Part model, mm, in its own coordinate system. A direction names the side the tool comes from. Round coordinates to 2 decimals unless told otherwise and drop trailing zeros. Write each question's results on one line, items separated by ' | '. Start each with the question number.
(1) Drill centre lines: L1, parallel to Z at x = 9.5, y = 10.15; L2, parallel to X at y = 7, z = 9.5; L3, parallel to X at y = -5.5, z = 13.25. Where is each one in solid material? Low to high.
(2) Tool access for faces 1 (the face through (7, 7, 24)), 2 (the face through (8.2, 3.5, 13.4)), 3 (the face through (5.137, -4.644, 14.37)), 4 (the face through (11.452, 11.451, 18.566)): list every direction of +Z, -Z, +X, -X, +Y, -Y with a clear straight run to the whole face (end or side of a thin tool).
(3) Flat gauge pins, fed straight in: P1, Ø6, axis at x = 9.5, z = 12, coming from the -Y side; P2, Ø5, axis at x = 0, y = 7, coming from the +Z side; P3, Ø2, axis at y = -5, z = 11, coming from the -X side; P4, Ø4, axis at x = 9.5, z = 12, coming from the -Y side. Where does each tip first touch, or does it go through?
(4) Mould opens along Y. For faces 5 (the face through (5.137, -1.856, 9.63)), 6 (the face through (-3.2, -8.5, 12.1)), 7 (the face through (11, 10, 12.8)), 8 (the face through (6, 14, 12)) say: released by +Y, released by -Y, zero draft, split by the parting line, or undercut.
(5) Cut at B-B, the plane x = -1.75. Give the number of separate pieces and of enclosed holes in the cut face, then the cut area to 3 significant figures.
Autodesk Inventor part; units mm, degrees
ref_plane "Work Plane1" through (7, 3.5, 17.0635) normal (0, 1, 0) x (1, 0, 0)
ref_plane "Work Plane3" through (0, 3.0314, 24) normal (1, 0, 0) x (0, 0, -1)
ref_plane "YZ Plane" through (0, 0, 0) normal (1, 0, 0) x (0, 1, 0)
sketch "Sketch1" plane through (0, 0, 0) normal (0, 0, 1) x (1, 0, 0)
  line L0 (0, 14) -> (0, 11)
  line L1 (0, 14) -> (15, 14)
  line L2 (15, 14) -> (15, 0)
  circle A0 centre (0, 7) radius 4
  line L3 (0, 3) -> (0, 0) construction
  line L4 (0, 0) -> (15, 0)
  line L5 (0, 11) -> (0, 3) construction
  line L6 (0.5, 0) -> (-0.5, 0)
  line L7 (-0.5, 0) -> (-0.5, 3.0314)
  line L8 (-0.5, 3.0314) -> (0.5, 3.0314)
  line L9 (0.5, 3.0314) -> (0.5, 0)
  line L10 (-0.5, 0) -> (-7, 0)
  line L11 (-7, 0) -> (-7, 14)
  line L12 (-7, 14) -> (0, 14)
  line L13 (-4, 10.1012) -> (-4, 3.4286) construction
  point P0 (0, 3.0314)
  dimension "d0" = 8
  dimension "d1" = 15
  dimension "d2" = 14
  dimension "d79" = 1
  dimension "d80" = 3
  dimension "d81" = 3
extrude "Extrusion1" add sketch "Sketch1" along normal blind 24 contours L1 L2 L4 L9 A0 L0 | L0 A0 L7 L10 L11 L12
sketch "Sketch2" plane through (15, 0, 0) normal (1, 0, 0) x (0, 0, -1)
  line L0 (-24, 0) -> (-24, 14)
  line L1 (0, 0) -> (0, 14)
  point P0 (-19, 7)
  point P1 (-5, 7)
  point P2 (-24, 7)
  dimension "d5" = 5
  dimension "d6" = 5
  dimension "d7" = 14
hole "Hole1" at (15, 7, 19) at (15, 7, 5) direction (-1, 0, 0) diameter 4 depth 8
sketch "Sketch4" plane through (0, 14, 0) normal (0, 1, 0) x (1, 0, 0)
  circle A0 centre (9.5, -5) radius 3.5
  circle A1 centre (9.5, -19) radius 3.5
  line L0 (15, -24) -> (-7, -24)
  line L1 (15, 0) -> (0, 0)
  line L2 (-0.5, 0) -> (0.5, 0)
  line L3 (-0.5, -24) -> (0.5, -24)
  line L4 (4, -24) -> (4, 0)
  line L5 (4, -24) -> (4, 0)
  line L6 (4, -24) -> (4, 0)
  line L7 (15, 0) -> (15, -24)
  line L8 (0.5, 0) -> (0.5, -24)
  line L9 (-0.5, 0) -> (-0.5, -24)
  point P0 (4, -24)
  point P1 (0, -24)
  dimension "d18" = 7
  dimension "d19" = 7
  dimension "d20" = 14
  dimension "d21" = 5
  dimension "d22" = 5
  dimension "d42" = 5.5
  dimension "d43" = 5.5
extrude "Extrusion2" add sketch "Sketch4" along normal blind 1 contours A0 | A1
sketch "Sketch3" plane through (2, 15, 0) normal (0, 1, 0) x (1, 0, 0)
  circle A0 centre (7.5, -5) radius 3.5
  circle A1 centre (7.5, -19) radius 3.5
hole "Hole2" at (9.5, 15, 19) at (9.5, 15, 5) direction (0, -1, 0) diameter 4 depth 7
sketch "Sketch5" plane through (15, 0, 0) normal (1, 0, 0) x (0, 0, -1)
  line L0 (-17.0635, 7.5) -> (-6.9365, 7.5)
  line L1 (-6.9365, 7.5) -> (-6.9365, 6.5)
  line L2 (-6.9365, 6.5) -> (-17.0635, 6.5)
  line L3 (-17.0635, 6.5) -> (-17.0635, 7.5)
  circle A0 centre (-5, 7) radius 2
  circle A1 centre (-19, 7) radius 2
  point P0 (0, 0)
  point P1 (-6.9365, 7)
  point P2 (-17.0635, 6.5)
  dimension "d35" = 1
extrude "Extrusion3" cut sketch "Sketch5" against normal blind 8 contours L0 A0 L2 A1
sketch "Sketch7" plane through (0, 14, 0) normal (0, 1, 0) x (1, 0, 0)
  circle A0 centre (9.5, -5) radius 2
  circle A1 centre (9.5, -19) radius 2
  point P0 (0, 0)
  point P1 (9.5, -12)
  dimension "d44" = 7
  dimension "d45" = 7
hole "Hole3" at (9.5, 14, 12) direction (0, -1, 0) diameter 3.4 end through all countersink diameter 6.3 countersink angle 90
chamfer "Chamfer3" distance 0.5 angle 45 2 edges at (15, 7, 21) (15, 7, 3)
ref_plane "Work Plane1" through (7, 3.5, 17.0635) normal (0, 1, 0) x (1, 0, 0)
sketch "Sketch10" plane through (7, 3.5, 17.0635) normal (0, 1, 0) x (1, 0, 0)
  circle A0 centre (2.5, 5.0635) radius 1.7
  line L0 (-0.25, 3.4758) -> (-0.25, 6.6512)
  line L1 (-0.25, 6.6512) -> (2.5, 8.2389)
  line L2 (2.5, 8.2389) -> (5.25, 6.6512)
  line L3 (5.25, 6.6512) -> (5.25, 3.4758)
  line L4 (5.25, 3.4758) -> (2.5, 1.8881)
  line L5 (2.5, 1.8881) -> (-0.25, 3.4758)
  point P0 (-7, 17.0635)
  dimension "d75" = 5.5
extrude "Extrusion6" cut sketch "Sketch10" against normal blind 10
sketch "Sketch12" plane through (-0.5, 0, 0) normal (1, 0, 0) x (0, 0, -1)
  circle A0 centre (-12, -3.25) radius 1.7
  circle A1 centre (-12, -3.25) radius 5.25
  line L0 (0, 0) -> (-8.616, -7.2639)
  line L1 (-24, 0) -> (-15.384, -7.2639)
  circle A2 centre (-12, -3.25) radius 3.25
  line L2 (0, 0) -> (-24, 0)
  point P0 (-12, 0)
  dimension "d82" = 3.4
  dimension "d84" = 2
  dimension "d95" = 6.5
extrude "Extrusion7" add sketch "Sketch12" against normal blind 5.5 contours A0 | A2 | A1 L2 | L1 L2 A1 | A1 L2 L0 picked at (-14.5812, -7.0055)
ref_plane "Work Plane3" through (0, 3.0314, 24) normal (1, 0, 0) x (0, 0, -1)
mirror "Mirror1" about plane through (0, 3.0314, 24) normal (1, 0, 0) of "Extrusion7"
fillet "Fillet1" radius 7 1 edges at (-7, 14, 12)
sketch "Sketch14" plane through (6.75, 3.5, 13.5877) normal (1, 0, 0) x (0, 0, -1)
  arc A0 (-1.7963, -10.7639) -> (4.9717, -10.7639) centre (1.5877, -6.75) ccw
  line L0 (0, -9.5) -> (-1.5877, -6.75)
  line L1 (-1.5877, -6.75) -> (0, -4)
  line L2 (0, -4) -> (3.1754, -4)
  line L3 (3.1754, -4) -> (4.7631, -6.75)
  line L4 (4.7631, -6.75) -> (3.1754, -9.5)
  line L5 (3.1754, -9.5) -> (0, -9.5)
  point P0 (13.5877, -3.5)
  dimension "d96" = 5.5
extrude "Extrusion8" cut sketch "Sketch14" against normal blind 2.5
sketch "Sketch13" plane through (-7, 0, 0) normal (-1, 0, 0) x (0, 0, 1)
  arc A0 (8.616, -7.2639) -> (15.384, -7.2639) centre (12, -3.25) ccw
  point P0 (0, 0)
hole "Hole4" at (-7, -3.25, 12) direction (1, 0, 0) diameter 3.4 end through all counterbore diameter 6.5 counterbore depth 3
sketch "Sketch15" plane through (0, 0, 24) normal (0, 0, 1) x (1, 0, 0)
  line L0 (6, 0) -> (15, 0)
  line L1 (15, 0) -> (15, 14)
  line L2 (14.5, 9) -> (14.5, 5)
  line L3 (15, 4.5) -> (15, 9.5)
  line L4 (6, 0) -> (15, 0)
  arc A0 (6, 0) -> (10.5, 1.125) centre (6, 9.5625) ccw
  line L5 (15, 0) -> (15, 14)
  arc A1 (15, 2.25) -> (10.5, 1.125) centre (15, -7.3125) ccw
  line L6 (15, 4.5) -> (15, 9.5)
  line L7 (15, 4.5) -> (15, 0)
  line L8 (15, 2.25) -> (10.6581, 2.25) construction
  point P0 (0, 0)
  point P1 (14.5, 6.5)
  point P2 (14.5, 7.5)
  point P3 (15, 7.5)
  point P4 (15, 6.5)
  point P5 (15, 2.25)
extrude "Extrusion9" cut sketch "Sketch15" against normal blind 28.75
chamfer "Chamfer5" distance 1 angle 45 13 edges at (0, 11, 24) (0, 11, 0) (-4.9497, 11.9497, 0) (-7, 3.5, 0) (7.5, 14, 0) (7.5, 14, 24) (-4.9497, 11.9497, 24) (-7, 3.5, 24) (-7, 0, 12) (8.3192, 0.2855, 0) (12.6808, 1.9645, 0) (12.6808, 1.9645, 24) (8.3192, 0.2855, 24)
chamfer "Chamfer6" distance 0.5 angle 45 2 edges at (6, 15, 19) (6, 15, 5)
equation "\"d81\" = d80"
equation "\"d22\" = d21"
equation "\"d42\" = d43"
properties part number "XY Joiner"
A:
1) L1: 0 to 3, 7 to 10.3, 13.7 to 17, 21 to 24 | L2: -7 to -4, 4 to 7 | L3: -4 to -0.5, 0.5 to 4.25
2) face 1: +Z, +X, -X, +Y, -Y | face 2: -Y | face 3: +X | face 4: +Y
3) P1: y = 0.01 | P2: through | P3: x = -4 | P4: y = 3.5
4) face 5: undercut | face 6: released by -Y | face 7: zero draft | face 8: released by +Y
5) separate pieces: 2 | enclosed holes: 1 | area: 263 mm2
